For this review, take the finished solid that the model builds, in its own axes (mm). A direction names the side the tool comes from. Round coordinates to 2 decimals unless told otherwise and drop trailing zeros. Order: outer loops, then holes, each group sorted by start corner. A loop starts at its lowest first (then second) coordinate and runs counter-clockwise, first axis right, second up. Notation, with made-up numbers: (17.25, -33.75) - (49.25, -33.75) arc R23 cw to (49.25, -24.75) - close; hole circle Ø11 at (-24.75, -0.75). An arc over 180 degrees is marked (long way). One line per item, written item: value.
```python
from build123d import *

# Parameters (mm, degrees)
SKETCH1_W           = 11
SKETCH1_H           = 12
BOSS_EXTRUDE1_DEPTH = 6
SKETCH2_W           = 8
SKETCH2_H           = 3
BOSS_EXTRUDE2_DEPTH = 6
SKETCH3_R           = 1.5
CUT_EXTRUDE1_DEPTH  = 6
SKETCH4_R           = 1.5
CUT_EXTRUDE2_DEPTH  = 16


with BuildPart() as part:
    # Sketch1 → Boss-Extrude1 (new body)
    with BuildSketch(Plane.XY):
        with Locations((5.5, 6)):
            Rectangle(SKETCH1_W, SKETCH1_H)
    extrude(amount=BOSS_EXTRUDE1_DEPTH)

    # Sketch2 → Boss-Extrude2 (add)
    with BuildSketch(Plane.XY.offset(6)):
        with Locations((7, 1.5)):
            Rectangle(SKETCH2_W, SKETCH2_H)
    extrude(amount=BOSS_EXTRUDE2_DEPTH)

    # Sketch3 → Cut-Extrude1 (cut)
    with BuildSketch(Plane(origin=(0, 3, 0), x_dir=(1, 0, 0), z_dir=(0, 1, 0))):
        with Locations((7, -9)):
            Circle(SKETCH3_R)
    extrude(amount=-CUT_EXTRUDE1_DEPTH, mode=Mode.SUBTRACT)

    # Sketch4 → Cut-Extrude2 (cut)
    with BuildSketch(Plane(origin=(0, 12, 0), x_dir=(1, 0, 0), z_dir=(0, 1, 0))):
        with Locations((7, -3)):
            Circle(SKETCH4_R)
    extrude(amount=-CUT_EXTRUDE2_DEPTH, mode=Mode.SUBTRACT)


solid = part.part
```
Item 1: Wall thickness on line 1 (Z direction, x = 7, y = 1); line 2 (X direction, y = 2.3, z = 9); line 3 (X direction, y = 8.25, z = 3): over which ranges is each line inside the solid? List them lowest first.
Returned:
line 1: 0 to 1.5, 4.5 to 7.5, 10.5 to 12
line 2: 3 to 5.5, 8.5 to 11
line 3: 0 to 5.5, 8.5 to 11
Item 2: The part is to be moulded in two halves that separate along X. For faces 1 (the flat face through (5, 7, 6)), 2 (the cylindrical face through (5.8, 1.5, 9.9)), 3 (the flat face through (3, 1, 9)), say which applies: +X half, -X half, draft (parallel to the pull), parting line (faces both ways), or undercut.
Returned:
face 1: draft
face 2: undercut
face 3: -X half
Item 3: Take a section at A-A (z = 3). Write out the cut boundary in (x, y), plus the area to 3 significant figures.
Returned:
outline: (0, 0) - (5.5, 0) - (5.5, 12) - (0, 12) - close; (8.5, 0) - (11, 0) - (11, 12) - (8.5, 12) - close
area: 96.0 mm^2
Item 4: Take a section at D-D (y = 7.25). Write out the cut boundary in (x, z), plus the area to 3 significant figures.
Returned:
outline: (0, 0) - (11, 0) - (11, 6) - (0, 6) - close; hole circle Ø3 at (7, 3)
area: 58.9 mm^2
Item 5: Take a section at C-C (y = 2.75). Write out the cut boundary in (x, z).
Returned:
outline: (0, 0) - (11, 0) - (11, 12) - (3, 12) - (3, 6) - (0, 6) - close; hole circle Ø3 at (7, 3); hole circle Ø3 at (7, 9)
Item 6: Take a section at B-B (x = 7). Write out the cut boundary in (y, z).
Returned:
outline: (0, 0) - (12, 0) - (12, 1.5) - (0, 1.5) - close; (0, 4.5) - (12, 4.5) - (12, 6) - (3, 6) - (3, 7.5) - (0, 7.5) - close; (0, 10.5) - (3, 10.5) - (3, 12) - (0, 12) - close
Item 7: For P1, Ø3.5, axis at x = 4.5, y = 9, coming from the +Z side; P2, Ø1.5, axis at y = 1.5, z = 10, coming from the -X side; P3, Ø2, axis at x = 5.5, z = 10, coming from the +Y side, all flat-tipped, find the tip position at first contact; note any pin that passes through.
Returned:
P1: z = 6
P2: x = 3
P3: y = 3
Item 8: Machinability: for faces 4 (the flat face through (6.1, 3, 7.6)), 5 (the flat face through (7, 2, 12)), which of the approach directions +Z, -Z, +X, -X, +Y, -Y give a long, thin tool a straight path to every point of the face, cutting with its end or side? Answer none if there is none.
Returned:
face 4: +Z, +X, -X, +Y
face 5: +Z, +X, -X, +Y, -Y
